Build history of the part. All positions in model axes, mm. A direction names the side the tool comes from. Give positions to 0.01 mm unless a question says otherwise; leave off trailing zeros. Order: outer loops, then holes, each group sorted by start corner. A loop starts at its lowest first (then second) coordinate and runs counter-clockwise, first axis right, second up. Notation, with made-up numbers: (78.5, -14) - (137.5, -14) arc R10 cw to (137.5, 2) - close; hole circle Ø7 at (37, 13). An arc over 180 degrees is marked (long way). Answer in a Markdown table with one row per item.
```python
from build123d import *

# Parameters (mm, degrees)
CROQUIS1_W              = 168
CROQUIS1_H              = 148.15
SALIENTE_EXTRUIR1_DEPTH = 5
CROQUIS2_W              = 2.5
CROQUIS2_H              = 10.2
CORTAR_EXTRUIR1_DEPTH   = 5
CROQUIS4_W              = 8
CROQUIS4_H              = 2.5
SALIENTE_EXTRUIR2_DEPTH = 5
SKETCH1_W               = 10.2
SKETCH1_H               = 2.5
CUT_EXTRUDE2_DEPTH      = 5


with BuildPart() as part:
    # Croquis1 → Saliente-Extruir1 (new body)
    with BuildSketch(Plane(origin=(0, 0, 0), x_dir=(1, 0, 0), z_dir=(0, 1, 0))):
        Rectangle(CROQUIS1_W, CROQUIS1_H)
    extrude(amount=SALIENTE_EXTRUIR1_DEPTH)

    # Croquis2 → Cortar-Extruir1 (cut)
    with BuildSketch(Plane(origin=(0, 5, 0), x_dir=(1, 0, 0), z_dir=(0, 1, 0))):
        with Locations((-81.5, 34.075)):
            Rectangle(CROQUIS2_W, CROQUIS2_H)
        with Locations((-81.5, -34.075)):
            Rectangle(CROQUIS2_W, CROQUIS2_H)
        with Locations((81.5, -34.075)):
            Rectangle(CROQUIS2_W, CROQUIS2_H)
        with Locations((81.5, 25)):
            Rectangle(CROQUIS2_W, CROQUIS2_H)
    extrude(amount=-CORTAR_EXTRUIR1_DEPTH, mode=Mode.SUBTRACT)

    # Croquis4 → Saliente-Extruir2 (add)
    with BuildSketch(Plane.XY.offset(74.075)):
        with Locations((-54, 2.5)):
            Rectangle(CROQUIS4_W, CROQUIS4_H)
        with Locations((54, 2.5)):
            Rectangle(CROQUIS4_W, CROQUIS4_H)
    extrude(amount=SALIENTE_EXTRUIR2_DEPTH)

    # Sketch1 → Cut-Extrude2 (cut)
    with BuildSketch(Plane(origin=(0, 5, 0), x_dir=(1, 0, 0), z_dir=(0, 1, 0))):
        with Locations((-44, 67.49891)):
            Rectangle(SKETCH1_W, SKETCH1_H)
        with Locations((44, 67.49891)):
            Rectangle(SKETCH1_W, SKETCH1_H)
    extrude(amount=-CUT_EXTRUDE2_DEPTH, mode=Mode.SUBTRACT)


solid = part.part
```
1. Cut at C-C on y = 2.95. Count the separate pieces of the cut face and the enclosed holes in it, and give its area (3 significant figures).
Check result:
| item | result |
|---|---|
| separate pieces | 1 |
| enclosed holes | 6 |
| area | 24,800 mm² |
2. Cut at A-A on x = -41.5. Write the cut outline in (y, z) (3 decimals).
Check result:
| item | result |
|---|---|
| outline | (0, -74.075) - (5, -74.075) - (5, -68.749) - (0, -68.749) - close; (0, -66.249) - (5, -66.249) - (5, 74.075) - (0, 74.075) - close |
3. Probe line 1 (X direction, y = 3.25, z = 36); line 2 (X direction, y = 2.45, z = -67.5); line 3 (X direction, y = 1.1, z = -22.5). List the from-to ranges inside material, lowest first.
Check result:
| item | result |
|---|---|
| line 1 | x = -84 to -82.75, -80.25 to 80.25, 82.75 to 84 |
| line 2 | x = -84 to -49.1, -38.9 to 38.9, 49.1 to 84 |
| line 3 | x = -84 to 80.25, 82.75 to 84 |
4. Two-plate mould, pull along X, no slides. Class faces 1 (the face through (44, 3, -66.249)), 2 (the face through (-54, 3.75, 77)), 3 (the face through (84, 2, 1)): +X half, -X half, draft (parallel to the pull), parting line (faces both ways), or undercut.
Check result:
| item | result |
|---|---|
| face 1 | undercut |
| face 2 | draft |
| face 3 | +X half |
5. Cut at D-D on x = 31. Write the cut outline in (y, z) (3 decimals), and give its area (3 significant figures).
Check result:
| item | result |
|---|---|
| outline | (0, -74.075) - (5, -74.075) - (5, 74.075) - (0, 74.075) - close |
| area | 741 mm² |
6. Which spindle directions (+Z, -Z, +X, -X, +Y, -Y) get a long thin tool onto all of the face, cutting with end or side? Do faces 4 (the face through (54, 3.75, 77)), 5 (the face through (-44, 3, -68.749)), 6 (the face through (54, 1.25, 77)). Say none if no direction does.
Check result:
| item | result |
|---|---|
| face 4 | +Z, +X, -X, +Y |
| face 5 | +Y, -Y |
| face 6 | +Z, +X, -X, -Y |
7. Drop flat-ended pins along their axis: P1, Ø2, axis at y = 3, z = 76.5, coming from the -X side; P2, Ø0.8, axis at y = 2.5, z = 76.5, coming from the +X side; P3, Ø1, axis at x = -37, y = 2, coming from the +Z side (3 decimals). Give the stop position or say it passes through.
Check result:
| item | result |
|---|---|
| P1 | stops at x = -58 |
| P2 | stops at x = 58 |
| P3 | stops at z = 74.075 |
8. Cut at B-B on x = 53. Write the cut outline in (y, z) (3 decimals).
Check result:
| item | result |
|---|---|
| outline | (0, -74.075) - (5, -74.075) - (5, 74.075) - (3.75, 74.075) - (3.75, 79.075) - (1.25, 79.075) - (1.25, 74.075) - (0, 74.075) - close |
